Autodesk Fusion 360 part; units mm, degrees
sketch "Sketch1" plane through (0, 0, 0) normal (0, 1, 0) x (1, 0, 0)
  circle A0 centre (0, 0) radius 12
  circle A1 centre (0, 0) radius 9.5 construction
  circle A2 centre (0, 0) radius 8 construction
  line L0 (0, 0) -> (0, -9.5) construction
  line L1 (0, 0) -> (0, 9.5) construction
  line L2 (0, 0) -> (8, 0) construction
  line L3 (0, 0) -> (-8, 0) construction
  circle A3 centre (0, 9.5) radius 1.5
  circle A4 centre (8, 0) radius 1.5
  circle A5 centre (-8, 0) radius 1.5
  circle A6 centre (0, 0) radius 2.5
  dimension "d1" = 24
  dimension "d2" = 19
  dimension "d3" = 16
  dimension "d5" = 3
  dimension "d6" = 3
  dimension "d7" = 3
  dimension "d10" = 5
extrude "Extrude1" add sketch "Sketch1" along normal blind 4.8
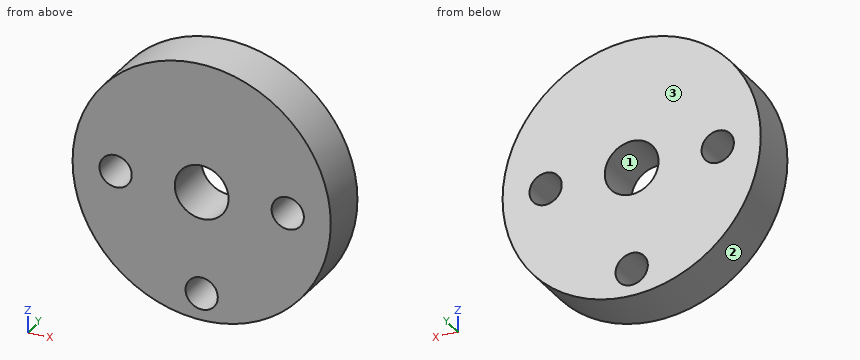
Verification items for the finished model (mm, model axes). Face numbers are marked on the shaded views. Give positions to 0.01 mm unless a question says otherwise; leave off trailing zeros. Write each loop counter-clockwise with the first axis right and the second up, starting at its lowest first coordinate (ties: lowest second). Pieces come first, ordered by that corner, then holes. Notation, with made-up numbers: M -13,-22.5 L 0,-22.5 A21 ccw 0,4.5 Z; hole C 40.5,22.25 d3. An arc over 180 degrees is marked long. Write item = value, one per line.
(1) Sectioned sample at C-C (x = -8.5). Record the cut outline in (y, z).
Found:
outline = M 0,-8.47 L 4.8,-8.47 L 4.8,-1.41 L 0,-1.41 Z; M 0,1.41 L 4.8,1.41 L 4.8,8.47 L 0,8.47 Z
(2) Go/stop test with flat-tipped pins: pin 1 Ø1.5 at (x, y) = (0.5, 2.5) entering from -Z; pin 2 Ø2 at (x, y) = (8, 4) entering from -Z; pin 3 Ø2 at (y, z) = (4, -2) entering from +X. Record where each tip stops, or that it passes through.
Found:
pin_1 = -12
pin_2 = -9.75
pin_3 = 11.96
(3) Sectioned sample at B-B (y = 3.6). Record the cut outline in (x, z).
Found:
outline = C 0,0 d24; hole C -8,0 d3; hole C 0,0 d5; hole C 0,-9.5 d3; hole C 8,0 d3
(4) Material ranges on line 1 (Z direction, x = 0, y = 3.45); line 2 (X direction, y = 3.6, z = 0); line 3 (X direction, y = 4.35, z = 0.5), recorded low to high.
Found:
line_1 = -12 to -11, -8 to -2.5, 2.5 to 12
line_2 = -12 to -9.5, -6.5 to -2.5, 2.5 to 6.5, 9.5 to 12
line_3 = -11.99 to -9.41, -6.59 to -2.45, 2.45 to 6.59, 9.41 to 11.99
(5) Sectioned sample at D-D (x = 8). Record the cut outline in (y, z), then the cut area to 3 significant figures.
Found:
outline = M 0,-8.94 L 4.8,-8.94 L 4.8,-1.5 L 0,-1.5 Z; M 0,1.5 L 4.8,1.5 L 4.8,8.94 L 0,8.94 Z
area = 71.5 mm2
(6) Draft check along Z on the marked faces 1, 2 and 3. Enter one of: released by +Z, released by -Z, zero draft, split by the parting line, or undercut.
Found:
face_1 = undercut
face_2 = split by the parting line
face_3 = zero draft
(7) Sectioned sample at A-A (x = 0). Record the cut outline in (y, z), then the cut area to 3 significant figures.
Found:
outline = M 0,-12 L 4.8,-12 L 4.8,-11 L 0,-11 Z; M 0,-8 L 4.8,-8 L 4.8,-2.5 L 0,-2.5 Z; M 0,2.5 L 4.8,2.5 L 4.8,12 L 0,12 Z
area = 76.8 mm2
